Check sheet for the modelled part. Datum: model origin and axes. Units: mm. Face numbers are marked on the shaded views. A direction names the side the tool comes from. Round coordinates to 2 decimals unless told otherwise and drop trailing zeros. Write each loop counter-clockwise with the first axis right and the second up, starting at its lowest first coordinate (ties: lowest second). Pieces come first, ordered by that corner, then holes. Notation, with made-up numbers: (65.5, -37) -> (111.5, -37) arc R13 ccw to (111.5, -26) -> close; hole circle Ø6 at (-13, -7.5). An arc over 180 degrees is marked (long way). One line per item, written item: value.
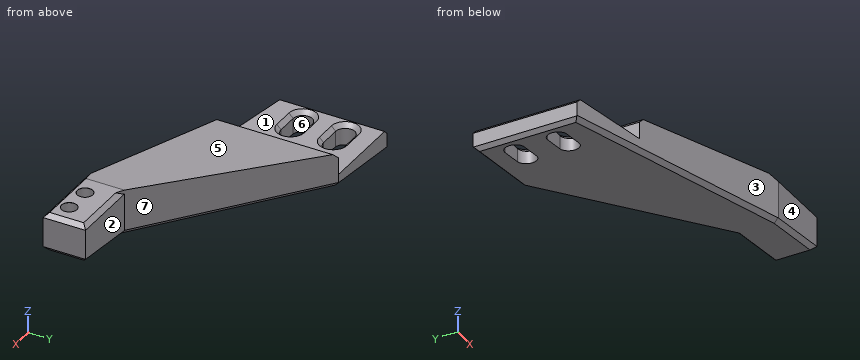
from build123d import *

# Parameters (mm, degrees)
BOSS_EXTRUDE1_DEPTH            = 18
CUT_EXTRUDE1_DEPTH             = 90.695930788
CHAMFER1_SIZE                  = 1
CHAMFER1_SIZE_2                = 1.13269448
CHAMFER1_SIZE_3                = 1.059024281
CHAMFER1_SIZE_4                = 0.982660718
CHAMFER1_SIZE_5                = 0.90514425
CHAMFER1_SIZE_6                = 1.228376825
M3_CLEARANCE_HOLE1_D           = 3.6
M3_CLEARANCE_HOLE1_DEPTH       = 4.418450886
M3_CLEARANCE_HOLE1_CSINK_D     = 3.65
M3_CLEARANCE_HOLE1_CSINK_ANGLE = 90
M3_CLEARANCE_HOLE1_TIP         = 1.081549114


with BuildPart() as part:
    # Sketch1 → Boss-Extrude1 (new body)
    with BuildSketch(Plane.XY):
        Polygon((0, 0), (0, 24.5), (64.6, 35), (80.6, 35), (80.6, 25), (64.6, 25), (20, 0), align=None)
        with BuildLine():
            Line((4.5, 19.5), (9.5, 19.5))
            ThreePointArc((9.5, 19.5), (11.75, 17.25), (9.5, 15))
            Line((9.5, 15), (4.5, 15))
            ThreePointArc((4.5, 15), (2.25, 17.25), (4.5, 19.5))
        make_face(mode=Mode.SUBTRACT)
        with BuildLine():
            Line((4.5, 9.5), (9.5, 9.5))
            ThreePointArc((9.5, 9.5), (11.75, 7.25), (9.5, 5))
            Line((9.5, 5), (4.5, 5))
            ThreePointArc((4.5, 5), (2.25, 7.25), (4.5, 9.5))
        make_face(mode=Mode.SUBTRACT)
    extrude(amount=BOSS_EXTRUDE1_DEPTH)

    # Sketch2 → Cut-Extrude1 (cut, through all)
    with BuildSketch(Plane.XZ):
        Polygon((0, 5.251895463), (20, 5.251895463), (20, 10.251895463), (64.6, 18), (0, 18), align=None)
        Polygon((0, 0), (80.6, 9), (80.6, 0), align=None)
    extrude(amount=-CUT_EXTRUDE1_DEPTH, mode=Mode.SUBTRACT)

    # Chamfer1
    # the kernel refuses this chamfer: 1.228376825, 1.13269448, 1.059024281, 1, 0.982660718, 0.90514425 mm, written as the material it takes off along each edge
    with BuildSketch(Plane(origin=(83.171682988, 25, 18), x_dir=(0, 0, -1), z_dir=(-1, 0, 0))) as chamfer1_piece_1_section:
        Polygon((CHAMFER1_SIZE, 0), (0, -CHAMFER1_SIZE), (0, 0), align=None)
    chamfer1_piece_1 = extrude(amount=26.286731952, mode=Mode.PRIVATE)
    chamfer1_piece_1 = split(chamfer1_piece_1, bisect_by=Plane(origin=(78.731517938, 32.921254449, 18), z_dir=(0.4889606682714293, -0.87230583219623, 0)), keep=Keep.TOP, mode=Mode.PRIVATE)
    add(chamfer1_piece_1, mode=Mode.SUBTRACT)
    with BuildSketch(Plane(origin=(80.6, 37.571682988, 18), x_dir=(0, 0, -1), z_dir=(0, -1, 0))) as chamfer1_piece_2:
        Polygon((CHAMFER1_SIZE, 0), (0, -CHAMFER1_SIZE), (0, 0), align=None)
    extrude(amount=15.143365976, mode=Mode.SUBTRACT)
    with BuildSketch(Plane(origin=(56.884951036, 35, 18), x_dir=(0, 0, -1), z_dir=(1, 0, 0))) as chamfer1_piece_3:
        Polygon((CHAMFER1_SIZE, 0), (0, -CHAMFER1_SIZE), (0, 0), align=None)
    extrude(amount=26.286731952, mode=Mode.SUBTRACT)
    with BuildSketch(Plane(origin=(9.5, 9.5, 5.251895463), x_dir=(0, 1, 0), z_dir=(-1, 0, 0)), Plane(origin=(4.5, 15, 5.251895463), x_dir=(0, -1, 0), z_dir=(1, 0, 0)), Plane(origin=(9.5, 19.5, 5.251895463), x_dir=(0, 1, 0), z_dir=(-1, 0, 0)), Plane(origin=(4.5, 5, 5.251895463), x_dir=(0, -1, 0), z_dir=(1, 0, 0))) as chamfer1_piece_4:
        Polygon((CHAMFER1_SIZE, 0), (0, CHAMFER1_SIZE), (0, 0), align=None)
    extrude(amount=5, mode=Mode.SUBTRACT)
    with BuildSketch(Plane(origin=(0, -2.571682988, 5.251895463), x_dir=(0, 0, -1), z_dir=(0, 1, 0))) as chamfer1_piece_5:
        Polygon((CHAMFER1_SIZE, 0), (0, -CHAMFER1_SIZE), (0, 0), align=None)
    extrude(amount=29.643365976, mode=Mode.SUBTRACT)
    with BuildSketch(Plane(origin=(4.5, 17.25, 5.251895463), x_dir=(0, -1, 0), z_dir=(1, 0, 0))) as chamfer1_piece_6:
        Polygon((2.25 + CHAMFER1_SIZE, 0), (2.25, CHAMFER1_SIZE), (2.25, 0), align=None)
    revolve(axis=Axis((4.5, 17.25, 5.251895463), (0, 0, -1)), revolution_arc=180, mode=Mode.SUBTRACT)
    with BuildSketch(Plane(origin=(9.5, 17.25, 5.251895463), x_dir=(0, 1, 0), z_dir=(-1, 0, 0))) as chamfer1_piece_7:
        Polygon((2.25 + CHAMFER1_SIZE, 0), (2.25, CHAMFER1_SIZE), (2.25, 0), align=None)
    revolve(axis=Axis((9.5, 17.25, 5.251895463), (0, 0, -1)), revolution_arc=180, mode=Mode.SUBTRACT)
    with BuildSketch(Plane(origin=(4.5, 7.25, 5.251895463), x_dir=(0, -1, 0), z_dir=(1, 0, 0))) as chamfer1_piece_8:
        Polygon((2.25 + CHAMFER1_SIZE, 0), (2.25, CHAMFER1_SIZE), (2.25, 0), align=None)
    revolve(axis=Axis((4.5, 7.25, 5.251895463), (0, 0, -1)), revolution_arc=180, mode=Mode.SUBTRACT)
    with BuildSketch(Plane(origin=(9.5, 7.25, 5.251895463), x_dir=(0, 1, 0), z_dir=(-1, 0, 0))) as chamfer1_piece_9:
        Polygon((2.25 + CHAMFER1_SIZE, 0), (2.25, CHAMFER1_SIZE), (2.25, 0), align=None)
    revolve(axis=Axis((9.5, 7.25, 5.251895463), (0, 0, -1)), revolution_arc=180, mode=Mode.SUBTRACT)
    with BuildSketch(Plane(origin=(80.6, 22.078920721, 9), x_dir=(-0.9938234393712555, 0, -0.11097284062458136), z_dir=(0, 1, 0))) as chamfer1_piece_10:
        Polygon((CHAMFER1_SIZE_2, 0), (-CHAMFER1_SIZE * 0.110972840625, CHAMFER1_SIZE * 0.993823439371), (0, 0), align=None)
    extrude(amount=15.842158559, mode=Mode.SUBTRACT)
    with BuildSketch(Plane(origin=(17.632153336, -1.327268309, 1.968850869), x_dir=(-0.48365166299246226, 0.873592837550041, -0.05400576882050032), z_dir=(0.8681970384240761, 0.48665753274892154, 0.09694507873221696))) as chamfer1_piece_11_section:
        Polygon((CHAMFER1_SIZE, 0), (-CHAMFER1_SIZE_3 * 0.0542613542965, CHAMFER1_SIZE_3 * 0.998526767225), (0, 0), align=None)
    chamfer1_piece_11 = extrude(amount=56.825456831, mode=Mode.PRIVATE)
    chamfer1_piece_11 = split(chamfer1_piece_11, bisect_by=Plane(origin=(17.632153336, 25, 1.968850869), z_dir=(0, -1, 0)), keep=Keep.TOP, mode=Mode.PRIVATE)
    add(chamfer1_piece_11, mode=Mode.SUBTRACT)
    with BuildSketch(Plane(origin=(72.169278028, 36.230300608, 8.058604246), x_dir=(0.15848267298847146, -0.987203157180204, 0.017696576388291016), z_dir=(-0.9811056370269924, -0.15946763450129123, -0.10955273862584283))) as chamfer1_piece_12:
        Polygon((CHAMFER1_SIZE, 0), (CHAMFER1_SIZE_4 * 0.0178037373512, CHAMFER1_SIZE_4 * 0.999841500402), (0, 0), align=None)
    extrude(amount=76.130813937, mode=Mode.SUBTRACT)
    with BuildSketch(Plane(origin=(0, -2.571682988, 0), x_dir=(0, 0, 1), z_dir=(0, 1, 0))) as chamfer1_piece_13:
        Polygon((CHAMFER1_SIZE_5, 0), (CHAMFER1_SIZE * 0.110972840625, CHAMFER1_SIZE * 0.993823439371), (0, 0), align=None)
    extrude(amount=29.643365976, mode=Mode.SUBTRACT)
    with BuildSketch(Plane(origin=(20, -3.172174758, 10.251895463), x_dir=(0.9852431265776485, 0, 0.17116068921192124), z_dir=(0, 1, 0))) as chamfer1_piece_14:
        Polygon((CHAMFER1_SIZE_6, 0), (-CHAMFER1_SIZE * 0.171160689212, CHAMFER1_SIZE * 0.985243126578), (0, 0), align=None)
    extrude(amount=34.095123509, mode=Mode.SUBTRACT)
    # the kernel refuses this chamfer: 1.228376825, 1.13269448, 1.059024281, 1, 0.982660718, 0.90514425 mm, written as the material it takes off along each edge
    with BuildSketch(Plane(origin=(-1.561975393, 0, -0.174414126), x_dir=(-0.11097284062458186, 0, 0.9938234393712553), z_dir=(0.9938234393712554, 0, 0.11097284062458188))) as chamfer1_2_piece_1:
        Polygon((CHAMFER1_SIZE, 0), (0, -CHAMFER1_SIZE), (0, 0), align=None)
    extrude(amount=22.212831842, mode=Mode.SUBTRACT)
    with BuildSketch(Plane(origin=(82.030100508, 25, 9.159688642), x_dir=(-0.11097284062458178, -3.5527136788004942e-15, 0.9938234393712553), z_dir=(-0.9938234393712554, 0, -0.11097284062458179))) as chamfer1_2_piece_2_section:
        Polygon((CHAMFER1_SIZE, 0), (0, CHAMFER1_SIZE), (0, 0), align=None)
    chamfer1_2_piece_2 = extrude(amount=22.164943744, mode=Mode.PRIVATE)
    chamfer1_2_piece_2 = split(chamfer1_2_piece_2, bisect_by=Plane(origin=(79.195166365, 29.16494468, 13.640367099), z_dir=(0.42046301876729836, -0.6177234194276358, -0.6645514479253808)), keep=Keep.TOP, mode=Mode.PRIVATE)
    add(chamfer1_2_piece_2, mode=Mode.SUBTRACT)
    with BuildSketch(Plane(origin=(82.030100508, 35, 9.159688642), x_dir=(-0.11097284062458186, -7.105427357601003e-15, 0.9938234393712553), z_dir=(-0.9938234393712554, 0, -0.11097284062458188))) as chamfer1_2_piece_3:
        Polygon((CHAMFER1_SIZE, 0), (0, -CHAMFER1_SIZE), (0, 0), align=None)
    extrude(amount=18.982611683, mode=Mode.SUBTRACT)

    # M3 Clearance Hole1
    with Locations(Plane.XY.offset(18)):
        with Locations((69.4, 31.5), (75.9, 31.5)):
            CounterSinkHole(M3_CLEARANCE_HOLE1_D / 2, M3_CLEARANCE_HOLE1_CSINK_D / 2, depth=M3_CLEARANCE_HOLE1_DEPTH, counter_sink_angle=M3_CLEARANCE_HOLE1_CSINK_ANGLE)
            with Locations((0, 0, -(M3_CLEARANCE_HOLE1_DEPTH + M3_CLEARANCE_HOLE1_TIP / 2))):  # 118° drill point
                Cone(0, M3_CLEARANCE_HOLE1_D / 2, M3_CLEARANCE_HOLE1_TIP, mode=Mode.SUBTRACT)


with BuildPart() as body_2:
    # Mirror2: mirrored copy
    add(part.part.mirror(Plane(origin=(20, 0, 18), x_dir=(0, 0, 1), z_dir=(0, 1, 0))))


solid = body_2.part
Item 1: Material ranges on line 1 along Y through (x, z) = (69.4, 16.3); line 2 along Y through (x, z) = (65.5, 13); line 3 along Z through (x, y) = (6, -20.5), recorded low to high.
Result set:
line 1: -35 to -33.3, -29.7 to -25
line 2: -35 to -25
line 3: 0.67 to 5.25
Item 2: Sectioned sample at B-B (y = -7.25). Enter the section's corners in (x, z), then the cut area to 3 significant figures.
Result set:
outline: (0, 0.91) -> (0.99, 0.11) -> (2.25, 0.25) -> (2.25, 4.25) -> (1.25, 5.25) -> (1, 5.25) -> (0, 4.25) -> close; (11.75, 1.31) -> (30.89, 3.45) -> (32.93, 4.74) -> (32.93, 12.5) -> (21.21, 10.46) -> (20, 9.25) -> (20, 5.25) -> (12.75, 5.25) -> (11.75, 4.25) -> close
area: 146 mm^2
Item 3: Tool access check on the marked faces 1, 2 and 3. Record the directions out of +Z, -Z, +X, -X, +Y, -Y that give a thin tool (end or side, any length) a straight path to the whole face; none if there is none.
Result set:
face 1: +Z, -X, +Y, -Y
face 2: +Z, -Z, +X, +Y
face 3: +Z, -Z, -X, -Y
Item 4: Depth check by flat-ended pin: pin 1 (5 mm diameter, centred on x = 52.5, z = 9.5, fed in from -Y); pin 2 (4 mm diameter, centred on x = 69.4, y = -31.5, fed in from -Z); pin 3 (5 mm diameter, centred on x = 42, z = 4.5, fed in from -Y). Enter the tip coordinate at first touch or a pass-through.
Result set:
pin 1: y = -33.44
pin 2: z = 7.53
pin 3: y = -31.66
Item 5: Sectioned sample at C-C (x = 23). Enter the section's corners in (y, z), then the cut area to 3 significant figures.
Result set:
outline: (-28.24, 3.56) -> (-27.23, 2.57) -> (-2.83, 2.57) -> (-1.68, 3.63) -> (-1.68, 10.77) -> (-28.24, 10.77) -> close
area: 217 mm^2
Item 6: Sectioned sample at A-A (x = 5.5). Enter the section's corners in (y, z).
Result set:
outline: (-25.39, 1.6) -> (-24.38, 0.61) -> (-19.5, 0.61) -> (-19.5, 4.25) -> (-20.5, 5.25) -> (-25.39, 5.25) -> close; (-15, 0.61) -> (-9.5, 0.61) -> (-9.5, 4.25) -> (-10.5, 5.25) -> (-14, 5.25) -> (-15, 4.25) -> close; (-5, 0.61) -> (-1, 0.61) -> (0, 1.62) -> (0, 5.25) -> (-4, 5.25) -> (-5, 4.25) -> close
Item 7: Sectioned sample at D-D (y = -17.25). Enter the section's corners in (x, z).
Result set:
outline: (0, 0.91) -> (0.99, 0.11) -> (2.25, 0.25) -> (2.25, 4.25) -> (1.25, 5.25) -> (1, 5.25) -> (0, 4.25) -> close; (11.75, 1.31) -> (48.73, 5.44) -> (50.77, 6.73) -> (50.77, 15.6) -> (21.21, 10.46) -> (20, 9.25) -> (20, 5.25) -> (12.75, 5.25) -> (11.75, 4.25) -> close
Item 8: Release check for a two-part mould opening along Y. For the marked faces 4, 5, 6 and 7 record: pulls with the +Y half, pulls with the -Y half, needs draft (parallel to the pull), parting line crosses it, or undercut.
Result set:
face 4: pulls with the -Y half
face 5: needs draft
face 6: undercut
face 7: pulls with the +Y half
